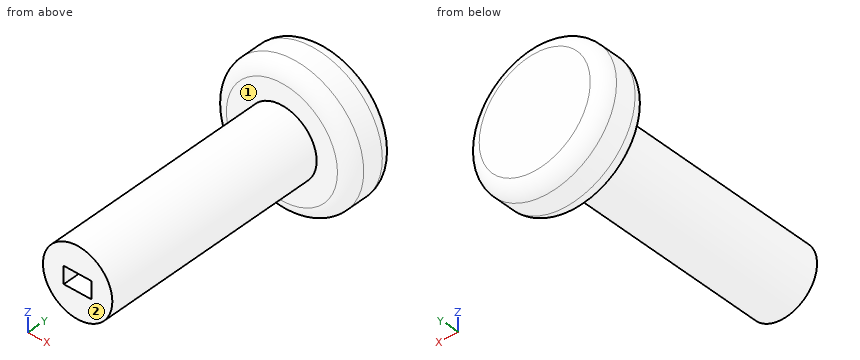
from build123d import *

# Parameters (mm, degrees)
SKETCH2_R           = 2.5
SKETCH2_W           = 2
SKETCH2_H           = 1.25
BOSS_EXTRUDE1_DEPTH = 10
FILLET1_R           = 1
SKETCH3_W           = 2
SKETCH3_H           = 1.25
BOSS_EXTRUDE5_DEPTH = 16
SKETCH4_R           = 5
THUMB_STICK_DEPTH   = 3.5
FILLET2_R           = 1
FILLET3_R           = 1


with BuildPart() as part:
    # Sketch2 → Boss-Extrude1 (new body, symmetric)
    with BuildSketch(Plane(origin=(0, 0, 0), x_dir=(1, 0, 0), z_dir=(0, 1, 0))):
        Circle(SKETCH2_R)
        Rectangle(SKETCH2_W, SKETCH2_H, mode=Mode.SUBTRACT)
    extrude(amount=BOSS_EXTRUDE1_DEPTH, both=True)

    # Fillet1
    fillet1_edges = [part.edges().sort_by_distance(p)[0] for p in [
        (-2.5, 10, 0),
    ]]
    fillet(fillet1_edges, radius=FILLET1_R)

    # Sketch3 → Boss-Extrude5 (add)
    with BuildSketch(Plane(origin=(0, 10, 0), x_dir=(1, 0, 0), z_dir=(0, 1, 0))):
        Rectangle(SKETCH3_W, SKETCH3_H)
    extrude(amount=-BOSS_EXTRUDE5_DEPTH)

    # Sketch4 → Thumb Stick (add)
    with BuildSketch(Plane(origin=(0, 10, 0), x_dir=(1, 0, 0), z_dir=(0, 1, 0))):
        Circle(SKETCH4_R)
    extrude(amount=-THUMB_STICK_DEPTH)

    # Fillet2
    fillet2_edges = [part.edges().sort_by_distance(p)[0] for p in [
        (-5, 6.5, 0),
    ]]
    fillet(fillet2_edges, radius=FILLET2_R)

    # Fillet3
    fillet3_edges = [part.edges().sort_by_distance(p)[0] for p in [
        (-5, 10, 0),
    ]]
    fillet(fillet3_edges, radius=FILLET3_R)


solid = part.part
Design review of the part built by this model. Coordinates are the model's own, in mm. Face numbers are marked on the shaded views. A direction names the side the tool comes from. Give positions to 0.01 mm unless a question says otherwise; leave off trailing zeros. Order: outer loops, then holes, each group sorted by start corner. A loop starts at its lowest first (then second) coordinate and runs counter-clockwise, first axis right, second up.
1. Add section D-D, the plane y = 1.75. State the section outline as (x, z) points.
Solution:
outline: circle Ø5 at (0, 0)
2. Add section A-A, the plane z = 0. State the section outline as (x, y) points, then the cut area to 3 significant figures.
Solution:
outline: (-5, 7.5) arc R1 ccw to (-4, 6.5) - (-2.5, 6.5) - (-2.5, -10) - (-1, -10) - (-1, -6) - (1, -6) - (1, -10) - (2.5, -10) - (2.5, 6.5) - (4, 6.5) arc R1 ccw to (5, 7.5) - (5, 9) arc R1 ccw to (4, 10) - (-4, 10) arc R1 ccw to (-5, 9) - close
area: 109 mm2
3. For pin 1 Ø1 at (y, z) = (-7.5, 0) entering from -X; pin 2 Ø4 at (x, y) = (1.5, 5.5) entering from -Z; pin 3 Ø1.4 at (y, z) = (-9, 0.5) entering from +X, all flat-tipped, find the tip position at first contact; note any pin that passes through.
Solution:
pin 1: stops at x = -2.5
pin 2: stops at z = -4.94
pin 3: stops at x = 2.5
4. Add section B-B, the plane y = -8.5. State the section outline as (x, z) points (3 decimals).
Solution:
outline: circle Ø5 at (0, 0); hole (-1, -0.625) - (1, -0.625) - (1, 0.625) - (-1, 0.625) - close
5. To check wall thickness, follow L1, parallel to Y at x = 2, z = 2.75; L2, parallel to X at y = -8.75, z = 0.25; L3, parallel to Y at x = -1.75, z = -4. State the ranges of each line that lie inside material, in increasing order.
Solution:
L1: y = 6.5 to 10
L2: x = -2.49 to -1, 1 to 2.49
L3: y = 6.57 to 9.93
6. Add section C-C, the plane x = 0. State the section outline as (y, z) points (3 decimals), then the cut area to 3 significant figures.
Solution:
outline: (-10, -2.5) - (6.5, -2.5) - (6.5, -4) arc R1 ccw to (7.5, -5) - (9, -5) arc R1 ccw to (10, -4) - (10, 4) arc R1 ccw to (9, 5) - (7.5, 5) arc R1 ccw to (6.5, 4) - (6.5, 2.5) - (-10, 2.5) - (-10, 0.625) - (-6, 0.625) - (-6, -0.625) - (-10, -0.625) - close
area: 112 mm2
7. Tool access review of the marked faces 1 and 2: name each direction out of +Z, -Z, +X, -X, +Y, -Y from which nothing blocks a thin tool from reaching the whole face with its end or side.
Solution:
face 1: -Y
face 2: +Z, -Z, +X, -X, -Y
